Model file for the job. Use its own axes, mm. Face numbers are marked on the shaded views. A direction names the side the tool comes from. Round coordinates to 2 decimals unless told otherwise and drop trailing zeros. Write each loop counter-clockwise with the first axis right and the second up, starting at its lowest first coordinate (ties: lowest second). Pieces come first, ordered by that corner, then holes.
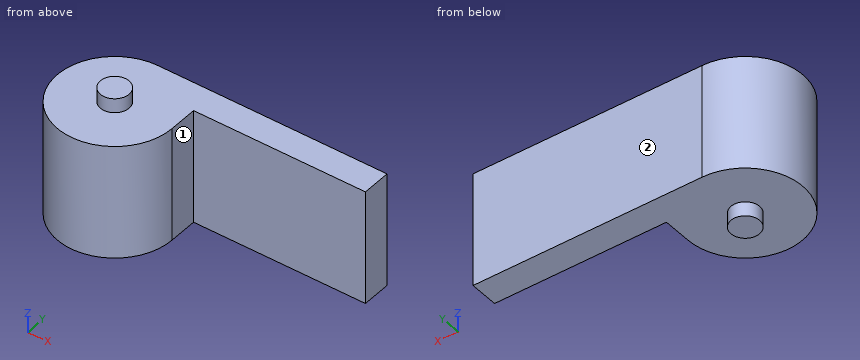
```python
from build123d import *

# Parameters (mm, degrees)
SKETCH1_R                = 6.35
SKETCH1_R_2              = 1.5875
BOSS_EXTRUDE1_DEPTH      = 12.7
BOSS_EXTRUDE2_DEPTH      = 14.2875
BOSS_EXTRUDE2_DEPTH_BACK = 1.5875
SKETCH1_3_R              = 1.5875


with BuildPart() as part:
    # Sketch1 → Boss-Extrude1 (new body)
    # profile 1 of 2: a face of its own
    with BuildSketch(Plane.XY):
        Circle(SKETCH1_R)
        Circle(SKETCH1_R_2, mode=Mode.SUBTRACT)
    # profile 2 of 2: a face of its own
    with BuildSketch(Plane.XY):
        with BuildLine():
            Line((25.4, 6.35), (0, 6.35))
            ThreePointArc((0, 6.35), (4.490128061, 4.490128061), (6.35, 0))
            Line((6.35, 0), (6.35, 3.175))
            Line((6.35, 3.175), (25.4, 3.175))
            Line((25.4, 3.175), (25.4, 6.35))
        make_face()
    extrude(amount=BOSS_EXTRUDE1_DEPTH)

    # Sketch1_3 → Boss-Extrude2 (add, two sides: drawn at the far end of the back side and taken through both)
    with BuildSketch(Plane.XY.offset(-BOSS_EXTRUDE2_DEPTH_BACK)):
        Circle(SKETCH1_3_R)
    extrude(amount=BOSS_EXTRUDE2_DEPTH + BOSS_EXTRUDE2_DEPTH_BACK)


solid = part.part
```
1) Cut at B-B on x = 17. List the corners of the cut face in (y, z) (3 decimals).
2) Wall check: probe 1 along Z at (x, y) = (-3, 1.25); probe 2 along Y at (x, z) = (19.5, 12.25) (3 decimals); probe 3 along X at (y, z) = (0.25, 9.5). Give the ranges that are in metal, low to high.
3) Flat gauge pins, fed straight in: pin 1 Ø5 at (x, z) = (5, 7) entering from -Y; pin 2 Ø6 at (x, y) = (17, 0.5) entering from -Z; pin 3 Ø1.5 at (x, y) = (4.5, -0.5) entering from +Z. Where does each tip first touch, or does it go through?
4) Cut at C-C on y = 5.5. List the corners of the cut face in (x, z).
5) Cut at A-A on z = 8. List the corners of the cut face in (x, y) (3 decimals).
6) Which spindle directions (+Z, -Z, +X, -X, +Y, -Y) get a long thin tool onto all of the face, cutting with end or side? Do the marked faces 1 and 2. Say none if no direction does.
Result sheet:
1. outline: (3.175, 0) - (6.35, 0) - (6.35, 12.7) - (3.175, 12.7) - close
2. probe 1: z = 0 to 12.7
2. probe 2: y = 3.175 to 6.35
2. probe 3: x = -6.35 to 6.35
3. pin 1: stops at y = -5.84
3. pin 2: stops at z = 0
3. pin 3: stops at z = 12.7
4. outline: (-3.17, 0) - (25.4, 0) - (25.4, 12.7) - (-3.17, 12.7) - close
5. outline: (0, 6.35) arc R6.35 ccw (long way) to (6.35, 0) - (6.35, 3.175) - (25.4, 3.175) - (25.4, 6.35) - close
6. face 1: +Z, -Z, +X, -Y
6. face 2: +Z, -Z, +X, -X, +Y
